For this review, take the finished solid that the model builds, in its own axes (mm). Coordinates: 2 decimals unless noted, no trailing zeros. Write each loop counter-clockwise with the first axis right and the second up, starting at its lowest first coordinate (ties: lowest second). Pieces come first, ordered by that corner, then holes. Notation, with made-up numbers: (29.5, 2.5) -> (84.5, 2.5) arc R22 ccw to (84.5, 38.5) -> close; hole circle Ø1 at (17, 68). An arc over 180 degrees is marked (long way). One line per item, written item: value. Start each with the question number.
1) Add section C-C (y = -5). State the section outline as (x, z) points, and give its area (3 significant figures).
2) Add section B-B (y = 2.5). State the section outline as (x, z) points.
3) Add section D-D (z = 0.85). State how many separate pieces and enclosed holes the cut face has, and give its area (3 significant figures).
4) Mouldability with a two-part tool opening along X and no side actions: class faces 1 (the cylindrical face through (6.87, 2.16, 1.48)), 2 (the flat face through (-7, 3, 0)), 3 (the cylindrical face through (-1.85, 14.08, 1.48)) as released by +X, released by -X, zero draft, split by the parting line, or undercut.
5) Add section A-A (x = 0). State the section outline as (y, z) points, and give its area (3 significant figures).
6) For probe 1 along Y at (x, z) = (0, 1); probe 2 along Y at (x, z) = (-5, 0.4); probe 3 along Y at (x, z) = (-9, 2.85), list the stretches that pass through material, from the lowest coordinate up. Write a range as from..to.
from build123d import *

# Parameters (mm, degrees)
F0_R     = 14.2
F0_R_2   = 7.2
F1_DEPTH = 3
F3_D     = 1
F5_D     = 0.5


with BuildPart() as f1:
    # F0 (on Top) → F1 (new body)
    with BuildSketch(Plane.XY):
        Circle(F0_R)
        Circle(F0_R_2, mode=Mode.SUBTRACT)
    extrude(amount=F1_DEPTH)

    # F3 (through all)
    with Locations(Plane.XY.offset(3)):
        with Locations((0, 10), (8.660254, 5), (8.660254, -5), (0, -10), (-8.660254, 5), (-8.660254, -5)):
            Hole(F3_D / 2)

    # F5 (through all)
    with Locations(Plane.XY.offset(3)):
        with Locations((-5, 8.660254), (5, 8.660254), (10, 0), (5, -8.660254), (-5, -8.660254), (-10, 0)):
            Hole(F5_D / 2)


solid = f1.part
Numbers:
1. outline: (-13.29, 0) -> (-9.16, 0) -> (-9.16, 3) -> (-13.29, 3) -> close; (-8.16, 0) -> (-5.18, 0) -> (-5.18, 3) -> (-8.16, 3) -> close; (5.18, 0) -> (8.16, 0) -> (8.16, 3) -> (5.18, 3) -> close; (9.16, 0) -> (13.29, 0) -> (13.29, 3) -> (9.16, 3) -> close
1. area: 42.7 mm²
2. outline: (-13.98, 0) -> (-6.75, 0) -> (-6.75, 3) -> (-13.98, 3) -> close; (6.75, 0) -> (13.98, 0) -> (13.98, 3) -> (6.75, 3) -> close
3. separate pieces: 1
3. enclosed holes: 13
3. area: 465 mm²
4. face 1: undercut
4. face 2: zero draft
4. face 3: split by the parting line
5. outline: (-14.2, 0) -> (-10.5, 0) -> (-10.5, 3) -> (-14.2, 3) -> close; (-9.5, 0) -> (-7.2, 0) -> (-7.2, 3) -> (-9.5, 3) -> close; (7.2, 0) -> (9.5, 0) -> (9.5, 3) -> (7.2, 3) -> close; (10.5, 0) -> (14.2, 0) -> (14.2, 3) -> (10.5, 3) -> close
5. area: 36.0 mm²
6. probe 1: -14.2..-10.5, -9.5..-7.2, 7.2..9.5, 10.5..14.2
6. probe 2: -13.29..-8.91, -8.41..-5.18, 5.18..8.41, 8.91..13.29
6. probe 3: -10.98..-5.37, -4.63..4.63, 5.37..10.98
